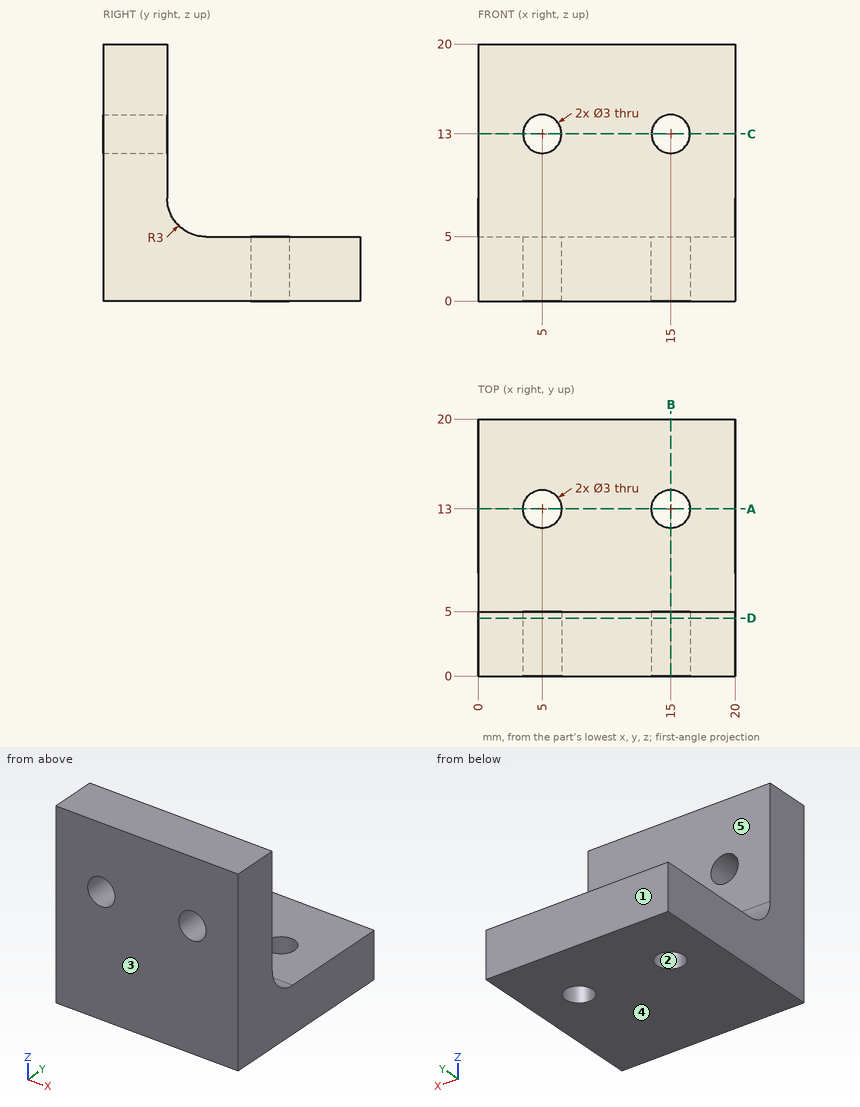
Design review of the part shown in the three views and the two pictorial views. Dimensions are in mm from the part's minimum x, y and z. A direction names the side the tool comes from. Give positions to 0.01 mm unless a question says otherwise; leave off trailing zeros. Loops run counter-clockwise (first coordinate to the right, second up) from the corner with the lowest first, then second, coordinate; pieces in that order, holes last. Notation, with made-up numbers: (44.25, 61.25) -> (56.25, 61.25) arc R11 ccw to (56.25, 72.25) -> close; hole circle Ø7 at (49, 4). An arc over 180 degrees is marked (long way). Write each question's results on one line, items separated by ' | '.
Q1. Take a section at A-A, the plane y = 13. Write out the cut boundary in (x, z).
Reply:
outline: (0, 0) -> (3.5, 0) -> (3.5, 5) -> (0, 5) -> close; (6.5, 0) -> (13.5, 0) -> (13.5, 5) -> (6.5, 5) -> close; (16.5, 0) -> (20, 0) -> (20, 5) -> (16.5, 5) -> close
Q2. Take a section at D-D, the plane y = 4.5. Write out the cut boundary in (x, z), plus the area to 3 significant figures.
Reply:
outline: (0, 0) -> (20, 0) -> (20, 20) -> (0, 20) -> close; hole circle Ø3 at (5, 13); hole circle Ø3 at (15, 13) | area: 386 mm²
Q3. Machinability: for the marked faces 4 and 5, which of the approach directions +Z, -Z, +X, -X, +Y, -Y give a long, thin tool a straight path to every point of the face, cutting with its end or side? Answer none if there is none.
Reply:
face 4: -Z, +X, -X, +Y, -Y | face 5: +Z, +X, -X, +Y
Q4. Take a section at B-B, the plane x = 15. Write out the cut boundary in (y, z).
Reply:
outline: (0, 0) -> (11.5, 0) -> (11.5, 5) -> (8, 5) arc R3 cw to (5, 8) -> (5, 11.5) -> (0, 11.5) -> close; (0, 14.5) -> (5, 14.5) -> (5, 20) -> (0, 20) -> close; (14.5, 0) -> (20, 0) -> (20, 5) -> (14.5, 5) -> close
Q5. The part is to be moulded in two halves that separate along Y. For the marked faces 1, 2 and 3, say which applies: +Y half, -Y half, draft (parallel to the pull), parting line (faces both ways), or undercut.
Reply:
face 1: +Y half | face 2: undercut | face 3: -Y half
Q6. For pin 1 Ø1.5 at (x, y) = (11.5, 16.5) entering from +Z; pin 2 Ø12 at (x, z) = (6, 13) entering from +Y; pin 3 Ø1 at (x, z) = (2.5, 17.5) entering from +Y, all flat-tipped, find the tip position at first contact; note any pin that passes through.
Reply:
pin 1: stops at z = 5 | pin 2: stops at y = 5.17 | pin 3: stops at y = 5
Q7. Wall thickness on L1, parallel to X at y = 2.7, z = 13; L2, parallel to Y at x = 15, z = 3.2; L3, parallel to Y at x = 4, z = 18: over which ranges is each line inside the solid? List them lowest first.
Reply:
L1: x = 0 to 3.5, 6.5 to 13.5, 16.5 to 20 | L2: y = 0 to 11.5, 14.5 to 20 | L3: y = 0 to 5
